Design review of the part built by this model. Coordinates are the model's own, in mm. A direction names the side the tool comes from. Coordinates: 2 decimals unless noted, no trailing zeros. Order: outer loops, then holes, each group sorted by start corner. A loop starts at its lowest first (then second) coordinate and runs counter-clockwise, first axis right, second up. Notation, with made-up numbers: (25, -14.5) -> (49, -14.5) arc R24 ccw to (49, 0.5) -> close; hole circle Ø8 at (5, -24.5). An arc over 180 degrees is marked (long way). Use a Markdown table: item, result. Add a question column.
Q1. Add section C-C (y = -55). State the section outline as (x, z) points.
Q2. Add section B-B (y = -32). State the section outline as (x, z) points.
Q3. Insertion check: pin 1 (8 mm diameter, centred on y = -66, z = -11, fed in from -X); pin 2 (5 mm diameter, centred on x = -36.5, z = -11, fed in from +Y); pin 3 (12 mm diameter, centred on y = -38, z = -4, fed in from +X); pin 4 (3 mm diameter, centred on y = -18.5, z = 3, fed in from -X). Each pin has a flat end and moves straight along its axis. Give the tip position at first contact, or say it passes through.
Q4. Add section D-D (y = -4). State the section outline as (x, z) points, then the cut area to 3 significant figures.
Q5. Machinability: for faces 1 (the face through (-25.07, -42.55, -1.12)), 2 (the face through (-47.745, -47.846, 2.253)), 3 (the face through (-25.07, -67.45, 1.12)), 4 (the face through (9.296, -77.465, -3.687)), 5 (the face through (-15.23, -45.46, 3)), which of the approach directions +Z, -Z, +X, -X, +Y, -Y give a long, thin tool a straight path to every point of the face, cutting with its end or side? Answer none if there is none.
Q6. The part is to be moulded in two halves that separate along Y. For faces 6 (the face through (-2, -20, 9)), 7 (the face through (-2.17, -0.14, -9.76)), 8 (the face through (-25.07, -47.805, 10.222)), 9 (the face through (-9, -25, 3)), say which applies: pulls with the +Y half, pulls with the -Y half, needs draft (parallel to the pull), parting line crosses it, or undercut.
Q7. Wall thickness on probe 1 along Y at (x, z) = (-7, -9); probe 2 along Z at (x, y) = (-52.5, -55); probe 3 along Y at (x, z) = (-50, 0): over which ranges is each line inside the solid? List them lowest first.
Q8. Add section A-A (x = -54). State the section outline as (y, z) points, then the cut area to 3 significant figures.
from build123d import *

# Parameters (mm, degrees)
F0_R      = 10
F1_DEPTH  = 10
F3_DEPTH  = 10
F4_R      = 9
F5_DEPTH  = 5
F6_R      = 12.5
F7_DEPTH  = 35
F8_R      = 15
F9_DEPTH  = 15
F10_R     = 1
F12_DEPTH = 5
F13_R     = 7.2112985608
F14_DEPTH = 2
F19_R     = 7.5
F19_R_2   = 6
F23_DEPTH = 10
F24_R     = 10
F25_DEPTH = 15


with BuildPart() as f1:
    # F0 (on Front) → F1 (new body, symmetric)
    with BuildSketch(Plane.XZ):
        Circle(F0_R)
    extrude(amount=F1_DEPTH, both=True)

    # F2 (on face) → F3 (join)
    with BuildSketch(Plane.XZ.offset(10)):
        Polygon((3.6354375365, -12.1703297922), (12.3575335407, -2.9367836356), (8.7220960043, 9.2335461566), (-3.6354375365, 12.1703297922), (-12.3575335407, 2.9367836356), (-8.7220960043, -9.2335461566), align=None)
    extrude(amount=F3_DEPTH)

    # F4 (on face) → F5 (join)
    with BuildSketch(Plane.XZ.offset(20)):
        Circle(F4_R)
    extrude(amount=F5_DEPTH)

    # F6 (on face) → F7 (join)
    with BuildSketch(Plane.XZ.offset(25)):
        Circle(F6_R)
    extrude(amount=F7_DEPTH)

    # F8 (on face) → F9 (join)
    with BuildSketch(Plane.XZ.offset(60)):
        Circle(F8_R)
    extrude(amount=F9_DEPTH)

    # F10
    f10_edges = [f1.edges().sort_by_distance(p)[0] for p in [
        (-15, -60, 0),
        (-12.5, -60, 0),
    ]]
    fillet(f10_edges, radius=F10_R)

    # F11 (on face) → F12 (join)
    with BuildSketch(Plane.XZ.offset(75)):
        Polygon((7.2396767244, -8.9955774834), (11.4102369845, 1.7719552168), (4.1705602602, 10.7675327002), (-7.2396767244, 8.9955774834), (-11.4102369845, -1.7719552168), (-4.1705602602, -10.7675327002), align=None)
    extrude(amount=F12_DEPTH)

    # F13 (on face) → F14 (join)
    with BuildSketch(Plane.XZ.offset(80)):
        Circle(F13_R)
    extrude(amount=F14_DEPTH)

    # F15 (on Right) → F16 (revolve)
    with BuildSketch(Plane.YZ):
        Polygon((-97, 0), (-82, 0), (-82, 7.2112985608), (-82, 15), (-97, 13), align=None)
    revolve(axis=Axis((0, -41, 0), (0, -1, 0)))

    # F19 (on offset) → F20 (join, up to the next surface of F1)
    with BuildSketch(Plane.YZ.offset(-65)):
        with Locations((-55, 0)):
            Circle(F19_R)
        with Locations((-55, 0)):
            Circle(F19_R_2, mode=Mode.SUBTRACT)
    extrude(until=Until.NEXT)

    # F22 (on offset) → F23 (join)
    with BuildSketch(Plane.YZ.offset(-30)):
        Polygon((-68.0466406272, -6.1740182765), (-56.1764636427, -14.3857313554), (-43.1298230155, -8.2117130789), (-41.9533593728, 6.1740182765), (-53.8235363573, 14.3857313554), (-66.8701769845, 8.2117130789), align=None)
    extrude(amount=F23_DEPTH)

    # F24 (on face) → F25 (join)
    with BuildSketch(Plane.YZ.offset(-20)):
        with Locations((-55, 0)):
            Circle(F24_R)
    extrude(amount=F25_DEPTH)


solid = f1.part
Established:
| question | item | result |
|---|---|---|
| 1 | outline | (-65, -7.5) -> (-30, -7.5) -> (-30, -13.83) -> (-20, -13.83) -> (-20, -10) -> (-7.5, -10) arc R12.5 ccw (long way) to (-7.5, 10) -> (-20, 10) -> (-20, 13.83) -> (-30, 13.83) -> (-30, 7.5) -> (-65, 7.5) -> (-65, 6) -> (-30, 6) -> (-30, -6) -> (-65, -6) -> close |
| 2 | outline | circle Ø25 at (0, 0) |
| 3 | pin 1 | x = -30 |
| 3 | pin 2 | through |
| 3 | pin 3 | x = 12.5 |
| 3 | pin 4 | x = -12.36 |
| 4 | outline | circle Ø20 at (0, 0) |
| 4 | area | 314 mm^2 |
| 5 | face 1 | -Z, -X, +Y |
| 5 | face 2 | -X |
| 5 | face 3 | +Z, -X, -Y |
| 5 | face 4 | -Z, +X |
| 5 | face 5 | none |
| 6 | face 6 | undercut |
| 6 | face 7 | needs draft |
| 6 | face 8 | pulls with the +Y half |
| 6 | face 9 | undercut |
| 7 | probe 1 | -97 to -82, -75 to -25, -20 to -10 |
| 7 | probe 2 | -7.5 to -6, 6 to 7.5 |
| 7 | probe 3 | -62.5 to -61, -49 to -47.5 |
| 8 | outline | circle Ø15 at (-55, 0); hole circle Ø12 at (-55, 0) |
| 8 | area | 63.6 mm^2 |
